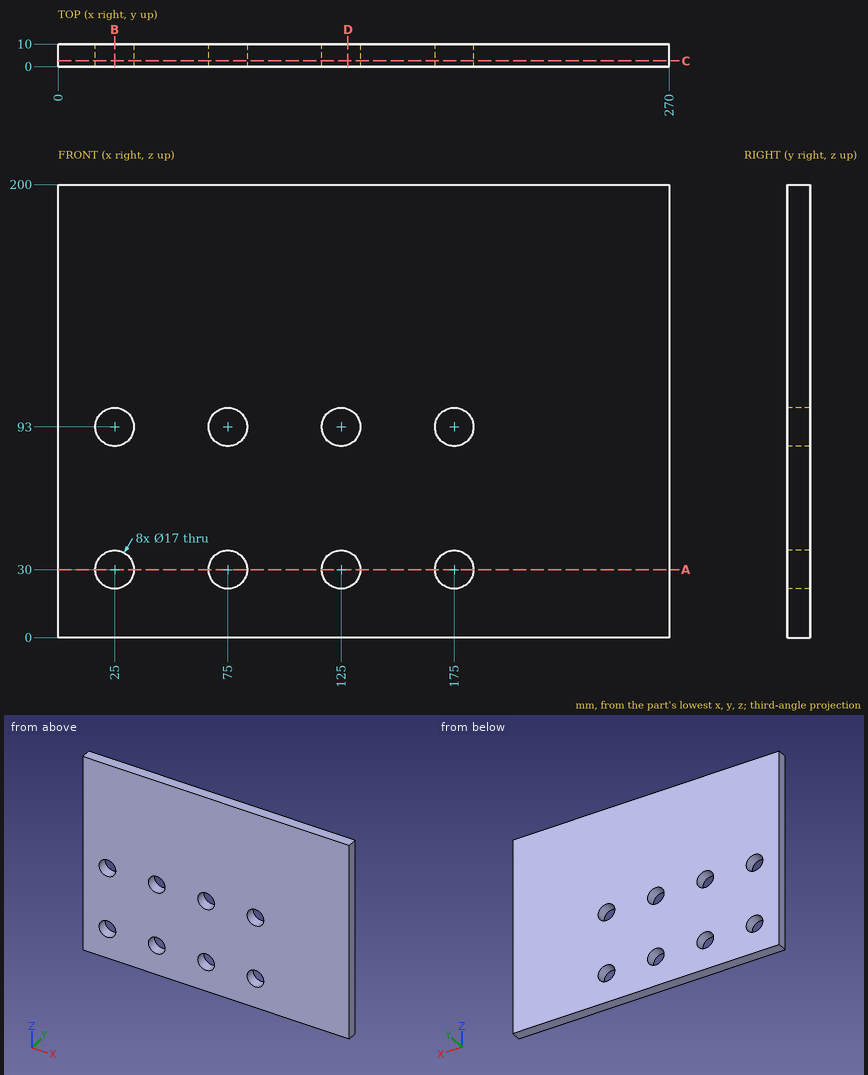
Print and shaded views of the part. All mm, measured from the part's lowest x, y and z. Round coordinates to 2 decimals unless told otherwise and drop trailing zeros. Write each loop counter-clockwise with the first axis right and the second up, starting at its lowest first coordinate (ties: lowest second). Pieces come first, ordered by that corner, then holes. Notation, with made-up numbers: (42, 88) - (93, 88) arc R9 ccw to (93, 99) - close; hole circle Ø4 at (-11.75, -7). An arc over 180 degrees is marked (long way). One line per item, written item: value.
(1) Cut at A-A, the plane z = 30. Give the cut face in (x, y).
Values follow:
outline: (0, 0) - (16.5, 0) - (16.5, 10) - (0, 10) - close; (33.5, 0) - (66.5, 0) - (66.5, 10) - (33.5, 10) - close; (83.5, 0) - (116.5, 0) - (116.5, 10) - (83.5, 10) - close; (133.5, 0) - (166.5, 0) - (166.5, 10) - (133.5, 10) - close; (183.5, 0) - (270, 0) - (270, 10) - (183.5, 10) - close
(2) Cut at B-B, the plane x = 25. Give the cut face in (y, z).
Values follow:
outline: (0, 0) - (10, 0) - (10, 21.5) - (0, 21.5) - close; (0, 38.5) - (10, 38.5) - (10, 84.5) - (0, 84.5) - close; (0, 101.5) - (10, 101.5) - (10, 200) - (0, 200) - close
(3) Cut at D-D, the plane x = 128. Give the cut face in (y, z), plus the area to 3 significant figures.
Values follow:
outline: (0, 0) - (10, 0) - (10, 22.05) - (0, 22.05) - close; (0, 37.95) - (10, 37.95) - (10, 85.05) - (0, 85.05) - close; (0, 100.95) - (10, 100.95) - (10, 200) - (0, 200) - close
area: 1,680 mm²
(4) Cut at C-C, the plane y = 2.5. Give the number of separate pieces and of enclosed holes in the cut face, plus the area to 3 significant figures.
Values follow:
separate pieces: 1
enclosed holes: 8
area: 52,200 mm²
(5) Wall check: probe 1 along Z at (x, y) = (25, 7.5). Give the ranges that are in metal, low to high.
Values follow:
probe 1: z = 0 to 21.5, 38.5 to 84.5, 101.5 to 200
